Geometry: final body of the model. Coordinates: model frame, mm. Round coordinates to 2 decimals unless told otherwise and drop trailing zeros. Loops run counter-clockwise (first coordinate to the right, second up) from the corner with the lowest first, then second, coordinate; pieces in that order, holes last. Notation, with made-up numbers: (-22.75, -5.75) - (33.25, -5.75) arc R28 ccw to (33.25, 13.25) - close; hole circle Ø1 at (30, 3.5). An arc over 180 degrees is marked (long way). Answer as CSV lines item,"result".
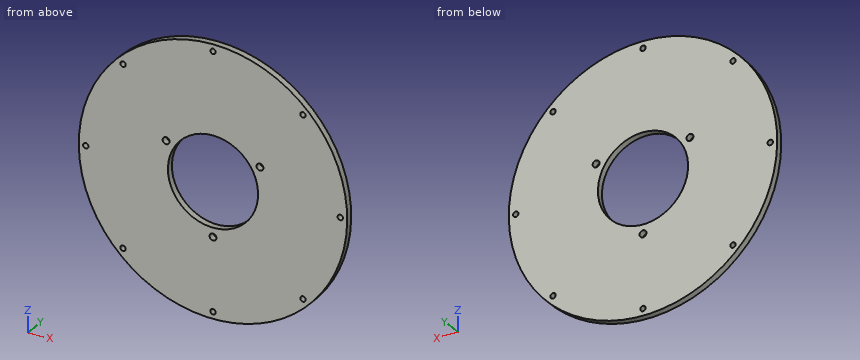
from build123d import *

# Parameters (mm, degrees)
SKETCH1_R           = 62.5
SKETCH1_R_2         = 21
BOSS_EXTRUDE1_DEPTH = 3.125
SKETCH2_R           = 1.6
CUT_EXTRUDE1_DEPTH  = 89.443573113
SKETCH6_R           = 1.25
CUT_EXTRUDE3_DEPTH  = 89.443573113


with BuildPart() as part:
    # Sketch1 → Boss-Extrude1 (new body)
    with BuildSketch(Plane(origin=(0, 0, 0), x_dir=(1, 0, 0), z_dir=(0, 1, 0))):
        with Locations(Location((0, 0, 0), (0, 0, 270))):
            Circle(SKETCH1_R)
        with Locations(Location((0, 0, 0), (0, 0, 270))):
            Circle(SKETCH1_R_2, mode=Mode.SUBTRACT)
    extrude(amount=BOSS_EXTRUDE1_DEPTH)

    # Sketch2 → Cut-Extrude1 (cut, through all)
    with BuildSketch(Plane(origin=(0, 3.125, 0), x_dir=(1, 0, 0), z_dir=(0, 1, 0))):
        with Locations(Location((0, 25.225, 0), (0, 0, 270))):
            Circle(SKETCH2_R)
        with Locations(Location((21.84549081, -12.6125, 0), (0, 0, 270))):
            Circle(SKETCH2_R)
        with Locations(Location((-21.84549081, -12.6125, 0), (0, 0, 270))):
            Circle(SKETCH2_R)
    extrude(amount=-CUT_EXTRUDE1_DEPTH, mode=Mode.SUBTRACT)

    # Sketch6 → Cut-Extrude3 (cut, through all)
    with BuildSketch(Plane(origin=(0, 3.125, 0), x_dir=(1, 0, 0), z_dir=(0, 1, 0))):
        with Locations(Location((-41.896076785, 41.896076785, 0), (0, 0, 270))):
            Circle(SKETCH6_R)
        with Locations(Location((41.896076785, 41.896076785, 0), (0, 0, 270))):
            Circle(SKETCH6_R)
        with Locations(Location((-41.896076785, -41.896076785, 0), (0, 0, 270))):
            Circle(SKETCH6_R)
        with Locations(Location((41.896076785, -41.896076785, 0), (0, 0, 270))):
            Circle(SKETCH6_R)
        with Locations(Location((-59.25, 0, 0), (0, 0, 270))):
            Circle(SKETCH6_R)
        with Locations(Location((59.25, 0, 0), (0, 0, 270))):
            Circle(SKETCH6_R)
        with Locations(Location((0, 59.25, 0), (0, 0, 270))):
            Circle(SKETCH6_R)
        with Locations(Location((0, -59.25, 0), (0, 0, 270))):
            Circle(SKETCH6_R)
    extrude(amount=-CUT_EXTRUDE3_DEPTH, mode=Mode.SUBTRACT)


solid = part.part
(1) Section C-C (x = -13). Output: boundary loops of the cut face in (y, z) (3 decimals), and give its area (3 significant figures).
Findings below:
outline,"(0, -61.133) - (3.125, -61.133) - (3.125, -16.492) - (0, -16.492) - close; (0, 16.492) - (3.125, 16.492) - (3.125, 61.133) - (0, 61.133) - close"
area,"279 mm2"
(2) Section B-B (y = 1.15). Give the number of separate pieces and of enclosed holes in the cut face, and give its area (3 significant figures).
Findings below:
separate pieces,"1"
enclosed holes,"12"
area,"10,800 mm2"
(3) Section D-D (z = -37.5). Output: boundary loops of the cut face in (x, y) (3 decimals).
Findings below:
outline,"(-50, 0) - (50, 0) - (50, 3.125) - (-50, 3.125) - close"
(4) Section A-A (z = -14.5). Output: boundary loops of the cut face in (x, y) (3 decimals).
Findings below:
outline,"(-60.795, 0) - (-15.19, 0) - (-15.19, 3.125) - (-60.795, 3.125) - close; (15.19, 0) - (60.795, 0) - (60.795, 3.125) - (15.19, 3.125) - close"
(5) Pin query (flat end, axial travel): P1, Ø3, axis at x = 59.25, z = 0, coming from the +Y side (3 decimals). Return the tip coordinate at first contact, or that it passes through.
Findings below:
P1,"y = 3.125"
(6) Material intervals for line 1 along X through (y, z) = (1.7, 0); line 2 along Z through (x, y) = (17.5, 1.4); line 3 along X through (y, z) = (1.5, 6), sorted ascending.
Findings below:
line 1,"-62.5 to -60.5, -58 to -21, 21 to 58, 60.5 to 62.5"
line 2,"-60 to -11.61, 11.61 to 60"
line 3,"-62.21 to -20.12, 20.12 to 62.21"
